Can you work these out from the drawing? Everything is in mm from the part's minimum corner. Give positions to 0.01 mm unless a question says otherwise; leave off trailing zeros. Order: outer loops, then holes, each group sorted by start corner. A loop starts at its lowest first (then second) coordinate and runs counter-clockwise, first axis right, second up. Notation, with made-up numbers: (49.25, 61.25) - (57.25, 61.25) arc R15 ccw to (57.25, 88.25) - close; hole circle Ø10 at (38, 43.5). An arc over 180 degrees is marked (long way). Answer as a JSON object with one key per item and string values.
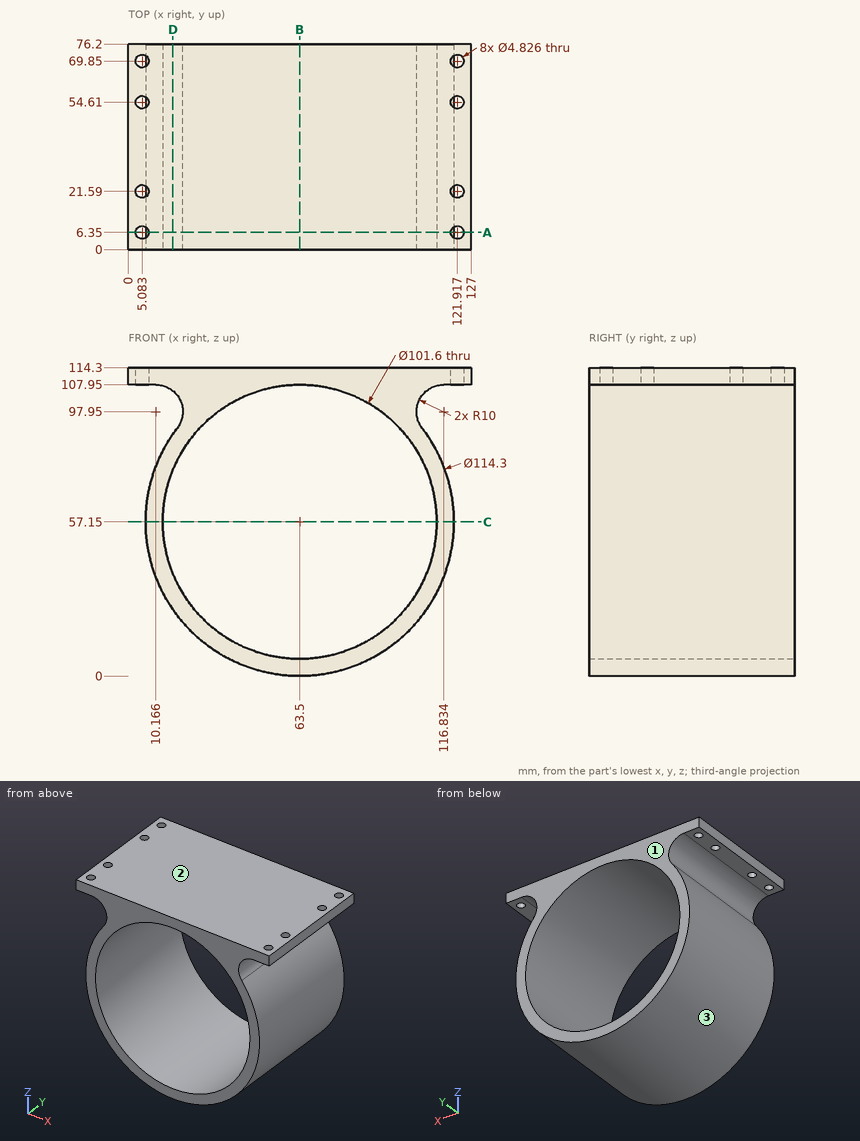
Q1. I'm going to push flat-ended pins straight in: pin 1 Ø2 at (y, z) = (13.5, 62.5) entering from +X; pin 2 Ø12 at (y, z) = (52, 76) entering from -X; pin 3 Ø7.5 at (x, y) = (5.08, 21.59) entering from +Z; pin 4 Ø4 at (y, z) = (63.5, 81) entering from +X. Where does each tip first touch, or does it pass through?
Recorded:
{"pin 1": "stops at x = 120.48", "pin 2": "stops at x = 7.81", "pin 3": "stops at z = 114.3", "pin 4": "stops at x = 116.31"}
Q2. We'd pull the mould along Z, two halves only. Please class the marked faces 1, 2 and 3: released by +Z, released by -Z, zero draft, split by the parting line, or undercut.
Recorded:
{"face 1": "zero draft", "face 2": "released by +Z", "face 3": "undercut"}
Q3. I need wall thicknesses on L1, parallel to X at y = 8, z = 58.5; L2, parallel to X at y = 6, z = 109 (1 decimal); L3, parallel to X at y = 46.5, z = 60. Which ranges of each line are inside material? Lowest first, please.
Recorded:
{"L1": "x = 6.37 to 12.72, 114.28 to 120.63", "L2": "x = 0 to 2.7, 7.5 to 119.5, 124.3 to 127", "L3": "x = 6.42 to 12.78, 114.22 to 120.58"}
Q4. If we section it at B-B, the plane x = 63.5: Please give me the cut outline in (y, z).
Recorded:
{"outline": "(0, 0) - (76.2, 0) - (76.2, 6.35) - (0, 6.35) - close; (0, 107.95) - (76.2, 107.95) - (76.2, 114.3) - (0, 114.3) - close"}
Q5. If we section it at C-C, the plane z = 57.15: Please give me the cut outline in (x, y).
Recorded:
{"outline": "(6.35, 0) - (12.7, 0) - (12.7, 76.2) - (6.35, 76.2) - close; (114.3, 0) - (120.65, 0) - (120.65, 76.2) - (114.3, 76.2) - close"}
Q6. If we section it at A-A, the plane y = 6.35: Please give me the cut outline in (x, z).
Recorded:
{"outline": "(0, 107.95) - (2.67, 107.95) - (2.67, 114.3) - (0, 114.3) - close; (7.5, 107.95) - (10.17, 107.95) arc R10 cw to (18.11, 91.87) arc R57.15 ccw (long way) to (108.89, 91.87) arc R10 cw to (116.83, 107.95) - (119.5, 107.95) - (119.5, 114.3) - (7.5, 114.3) - close; (124.33, 107.95) - (127, 107.95) - (127, 114.3) - (124.33, 114.3) - close; hole circle Ø101.6 at (63.5, 57.15)"}
Q7. If we section it at D-D, the plane x = 16.5: Please give me the cut outline in (y, z), then the cut area to 3 significant figures.
Recorded:
{"outline": "(0, 24.64) - (76.2, 24.64) - (76.2, 37.87) - (0, 37.87) - close; (0, 76.43) - (76.2, 76.43) - (76.2, 89.66) - (0, 89.66) - close; (0, 105.69) - (76.2, 105.69) - (76.2, 114.3) - (0, 114.3) - close", "area": "2,670 mm^2"}
